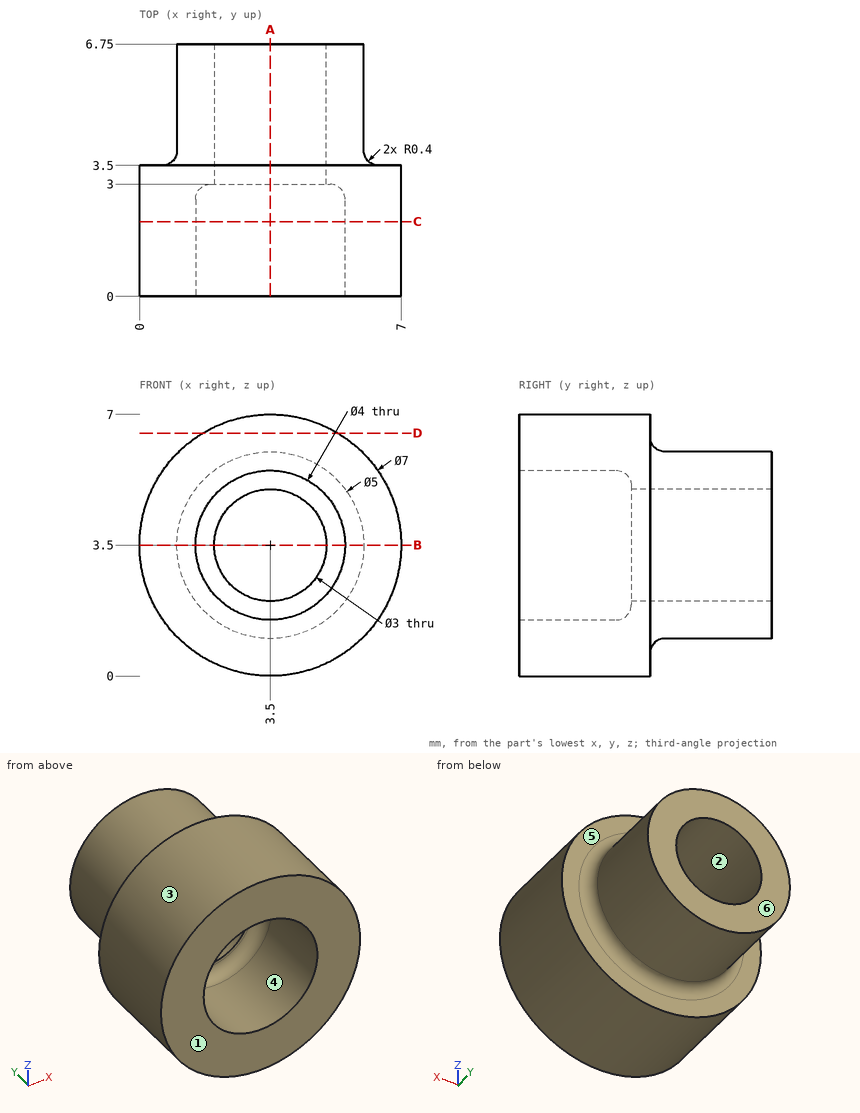
The figure shows three views and two pictorial views of one solid part (mm, origin at its lowest corner). Answer the questions. A direction names the side the tool comes from. Coordinates: 2 decimals unless noted, no trailing zeros. Write each loop counter-clockwise with the first axis right and the second up, starting at its lowest first coordinate (ties: lowest second). Pieces come first, ordered by that corner, then holes.
1. For the marked faces 5 and 6, determine the directions among +Z, -Z, +X, -X, +Y, -Y from which every point of the face is accessible in a straight line to the end or side of a thin tool.
Results list:
face 5: +Y
face 6: +Z, -Z, +X, -X, +Y
2. The part is cut by section D-D, the plane z = 6.5. Write down the section's boundary in (x, y), and give its area (3 significant figures).
Results list:
outline: (1.7, 0) - (5.3, 0) - (5.3, 3.5) - (1.7, 3.5) - close
area: 12.6 mm2
3. For a pull along Z with two mould halves and no side action, classify the marked faces 1, 2, 3 and 4 as +Z half, -Z half, draft (parallel to the pull), parting line (faces both ways), or undercut.
Results list:
face 1: draft
face 2: undercut
face 3: parting line
face 4: undercut
4. Flat-ended cylindrical pins translate along their axes: pin 1 (2 mm diameter, centred on x = 1, z = 1.5, fed in from -Y); pin 2 (1.5 mm diameter, centred on y = 3, z = 2.5, fed in from +X); pin 3 (1.5 mm diameter, centred on y = 2.5, z = 4.5, fed in from -X). Find the tip coordinate at first contact, or state that the pin passes through.
Results list:
pin 1: stops at y = 0
pin 2: stops at x = 6.99
pin 3: stops at x = 0.01
5. The part is cut by section A-A, the plane x = 3.5. Write down the section's boundary in (y, z).
Results list:
outline: (0, 0) - (3.5, 0) - (3.5, 0.6) arc R0.4 cw to (3.9, 1) - (6.75, 1) - (6.75, 2) - (3, 2) - (3, 1.9) arc R0.4 cw to (2.6, 1.5) - (0, 1.5) - close; (0, 5.5) - (2.6, 5.5) arc R0.4 cw to (3, 5.1) - (3, 5) - (6.75, 5) - (6.75, 6) - (3.9, 6) arc R0.4 cw to (3.5, 6.4) - (3.5, 7) - (0, 7) - close
6. The part is cut by section C-C, the plane y = 2. Write down the section's boundary in (x, z).
Results list:
outline: circle Ø7 at (3.5, 3.5); hole circle Ø4 at (3.5, 3.5)
7. Consider line 1 along X through (y, z) = (5.8, 3.5); line 2 along Z through (x, y) = (3.5, 2.05); line 3 along Z through (x, y) = (4.25, 2.5). Determine where each line is inside the solid, lowest interval first.
Results list:
line 1: x = 1 to 2, 5 to 6
line 2: z = 0 to 1.5, 5.5 to 7
line 3: z = 0.08 to 1.65, 5.35 to 6.92
8. The part is cut by section B-B, the plane z = 3.5. Write down the section's boundary in (x, y), and give its area (3 significant figures).
Results list:
outline: (0, 0) - (1.5, 0) - (1.5, 2.6) arc R0.4 cw to (1.9, 3) - (2, 3) - (2, 6.75) - (1, 6.75) - (1, 3.9) arc R0.4 cw to (0.6, 3.5) - (0, 3.5) - close; (5, 3) - (5.1, 3) arc R0.4 cw to (5.5, 2.6) - (5.5, 0) - (7, 0) - (7, 3.5) - (6.4, 3.5) arc R0.4 cw to (6, 3.9) - (6, 6.75) - (5, 6.75) - close
area: 17.6 mm2
